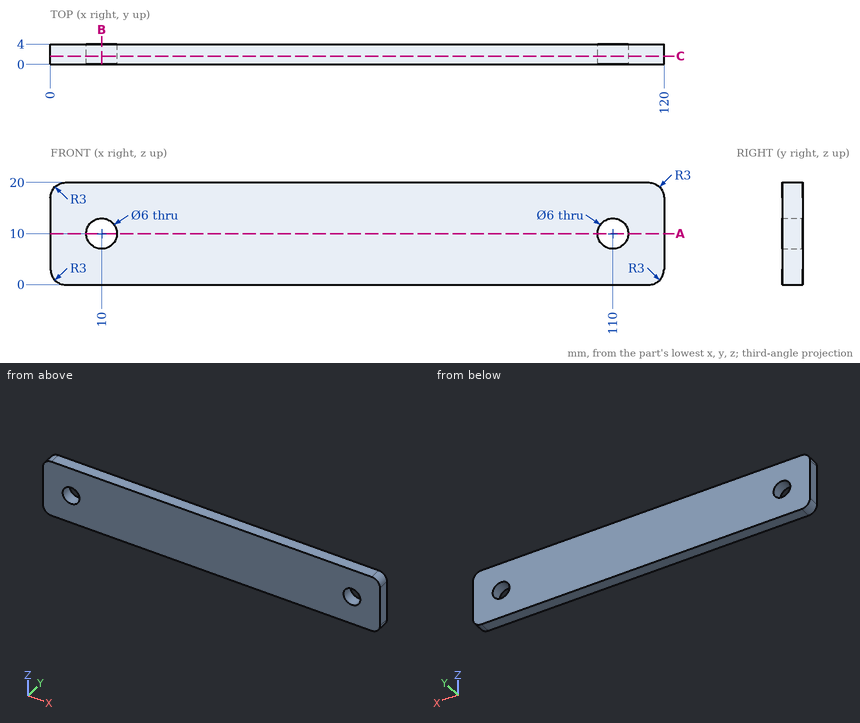
Job drawing, mm, ordinate dimensions from the low corner. One solid piece. Give positions to 0.01 mm unless a question says otherwise; leave off trailing zeros. Loops run counter-clockwise (first coordinate to the right, second up) from the corner with the lowest first, then second, coordinate; pieces in that order, holes last. Notation, with made-up numbers: M 8,5 L 61,5 A35 cw 61,39 Z; hole C -11,38 d8. An arc over 180 degrees is marked long. Answer in a Markdown table with one row per item. Add a question column.
Item 1: Drop a flat-ended pin along its axis: P1, Ø1.5, axis at x = 105, z = 7.5, coming from the -Y side. Give the stop position or say it passes through.
Item 2: Band-saw the part on B-B on x = 10. Give the cut face in (y, z), then the cut area to 3 significant figures.
Item 3: Band-saw the part on C-C on y = 1.65. Give the cut face in (x, z).
Item 4: Probe probe 1 along X at (y, z) = (2.45, 10); probe 2 along Z at (x, y) = (10, 2.4); probe 3 along X at (y, z) = (3.7, 11.25). List the from-to ranges inside material, lowest first.
Item 5: Band-saw the part on A-A on z = 10. Give the cut face in (x, y), then the cut area to 3 significant figures.
Reply:
| question | item | result |
|---|---|---|
| 1 | P1 | stops at y = 0 |
| 2 | outline | M 0,0 L 4,0 L 4,7 L 0,7 Z; M 0,13 L 4,13 L 4,20 L 0,20 Z |
| 2 | area | 56.0 mm^2 |
| 3 | outline | M 0,3 A3 ccw 3,0 L 117,0 A3 ccw 120,3 L 120,17 A3 ccw 117,20 L 3,20 A3 ccw 0,17 Z; hole C 10,10 d6; hole C 110,10 d6 |
| 4 | probe 1 | x = 0 to 7, 13 to 107, 113 to 120 |
| 4 | probe 2 | z = 0 to 7, 13 to 20 |
| 4 | probe 3 | x = 0 to 7.27, 12.73 to 107.27, 112.73 to 120 |
| 5 | outline | M 0,0 L 7,0 L 7,4 L 0,4 Z; M 13,0 L 107,0 L 107,4 L 13,4 Z; M 113,0 L 120,0 L 120,4 L 113,4 Z |
| 5 | area | 432 mm^2 |
